from build123d import *

# Parameters (mm, degrees)
SKETCH1_R           = 32.5
BOSS_EXTRUDE1_DEPTH = 12.5


with BuildPart() as part:
    # Sketch1 → Boss-Extrude1 (new body)
    # profile 1 of 2: a face of its own
    with BuildSketch(Plane(origin=(0, 0, 0), x_dir=(1, 0, 0), z_dir=(0, 1, 0))):
        with BuildLine():
            Line((0, -48), (10, -48))
            ThreePointArc((10, -48), (58, 0), (10, 48))
            Line((10, 48), (0, 48))
            Line((0, 48), (-50, 48))
            Line((-50, 48), (-50, -48))
            Line((-50, -48), (0, -48))
        make_face()
        with BuildLine():
            ThreePointArc((10, -40), (50, 0), (10, 40))
            Line((10, 40), (0, 40))
            Line((0, 40), (-42, 40))
            Line((-42, 40), (-42, -40))
            Line((-42, -40), (0, -40))
            Line((0, -40), (10, -40))
        make_face(mode=Mode.SUBTRACT)
    # profile 2 of 2: a face of its own
    with BuildSketch(Plane(origin=(0, 0, 0), x_dir=(1, 0, 0), z_dir=(0, 1, 0))):
        with BuildLine():
            Line((0, -40), (10, -40))
            ThreePointArc((10, -40), (50, 0), (10, 40))
            Line((10, 40), (0, 40))
            Line((0, 40), (-42, 40))
            Line((-42, 40), (-42, -40))
            Line((-42, -40), (0, -40))
        make_face()
        with Locations(Location((0, 0, 0), (0, 0, 270))):
            Circle(SKETCH1_R, mode=Mode.SUBTRACT)
    extrude(amount=BOSS_EXTRUDE1_DEPTH)


solid = part.part
The model under review builds one solid part; all positions refer to its coordinate system, in mm. Round coordinates to 2 decimals unless told otherwise and drop trailing zeros. Write each loop counter-clockwise with the first axis right and the second up, starting at its lowest first coordinate (ties: lowest second). Pieces come first, ordered by that corner, then holes. Notation, with made-up numbers: M -35.75,85.25 L -13.75,85.25 A16 cw -13.75,96.25 Z; hole C 44,47.5 d8. An arc over 180 degrees is marked long. Use a Markdown table: item, result. Add a question column.
Q1. We need section C-C, the plane y = 11.25. State the section outline as (x, z) points, plus the area to 3 significant figures.
Q2. Insertion check: pin 1 (10 mm diameter, centred on x = -11, z = -34, fed in from -Y); pin 2 (3 mm diameter, centred on x = 28.5, y = 9, fed in from -Z). Each pin has a flat end and moves straight along its axis. Give the tip position at first contact, or say it passes through.
Q3. The part is to be moulded in two halves that separate along X. For faces 1 (the face through (57.99, 6.16, 1.06)), 2 (the face through (9.76, 6.16, 31)), 3 (the face through (-20, 6, 48)), 4 (the face through (-50, 6, -1)), say which applies: pulls with the +X half, pulls with the -X half, needs draft (parallel to the pull), parting line crosses it, or undercut.
Q4. We need section B-B, the plane z = 0. State the section outline as (x, y) points, plus the area to 4 significant figures.
Q5. To check wall thickness, follow line 1 (X direction, y = 9.75, z = 0); line 2 (X direction, y = 3, z = -3); line 3 (Z direction, x = -5, y = 2.25). State the ranges of each line that lie inside material, in increasing order.
Q6. We need section D-D, the plane x = 49.5. State the section outline as (y, z) points, plus the area to 3 significant figures.
Q7. We need section A-A, the plane x = -16.5. State the section outline as (y, z) points, plus the area to 3 significant figures.
Findings below:
| question | item | result |
|---|---|---|
| 1 | outline | M -50,-48 L 10,-48 A48 ccw 10,48 L -50,48 Z; hole C 0,0 d65 |
| 1 | area | 6,060 mm² |
| 2 | pin 1 | stops at y = 0 |
| 2 | pin 2 | stops at z = -44.89 |
| 3 | face 1 | pulls with the +X half |
| 3 | face 2 | undercut |
| 3 | face 3 | needs draft |
| 3 | face 4 | pulls with the -X half |
| 4 | outline | M -50,0 L -32.5,0 L -32.5,12.5 L -50,12.5 Z; M 32.5,0 L 58,0 L 58,12.5 L 32.5,12.5 Z |
| 4 | area | 537.5 mm² |
| 5 | line 1 | x = -50 to -32.5, 32.5 to 58 |
| 5 | line 2 | x = -50 to -32.36, 32.36 to 57.91 |
| 5 | line 3 | z = -48 to -32.11, 32.11 to 48 |
| 6 | outline | M 0,-27.27 L 12.5,-27.27 L 12.5,27.27 L 0,27.27 Z |
| 6 | area | 682 mm² |
| 7 | outline | M 0,-48 L 12.5,-48 L 12.5,-28 L 0,-28 Z; M 0,28 L 12.5,28 L 12.5,48 L 0,48 Z |
| 7 | area | 500 mm² |
